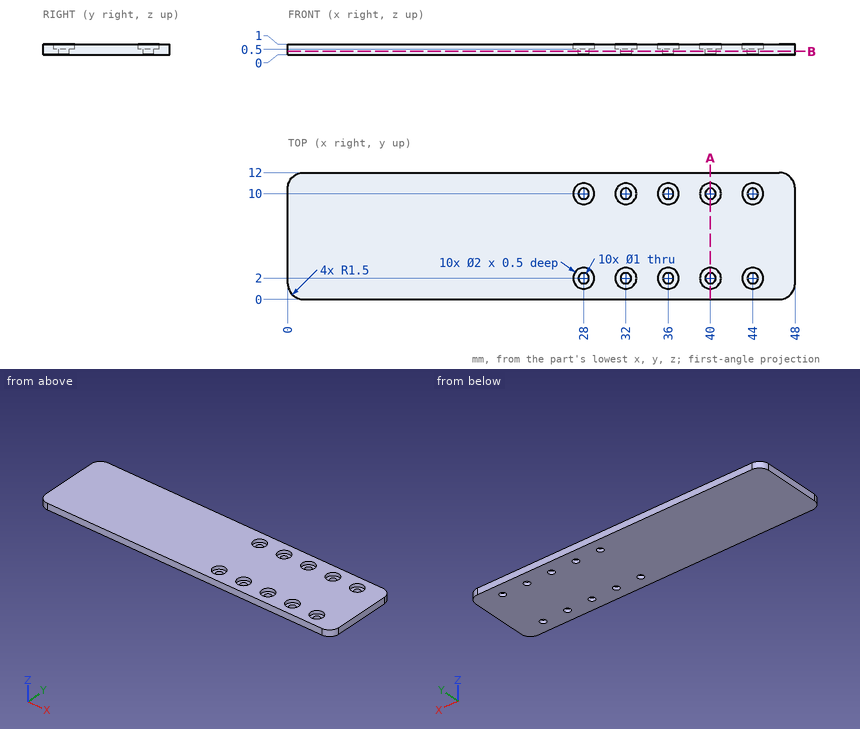
Study the drawing (mm; zero at the part's minimum x, y, z) and answer. Round coordinates to 2 decimals unless told otherwise and drop trailing zeros. Write each loop counter-clockwise with the first axis right and the second up, starting at its lowest first coordinate (ties: lowest second). Pieces come first, ordered by that corner, then holes. Notation, with made-up numbers: (78.5, 18.5) - (83.5, 18.5) arc R30 cw to (83.5, 55.5) - close; hole circle Ø4 at (-28.75, 11.5). An arc over 180 degrees is marked (long way). Return JSON: item names as keys, results as strings. Group by question number.
Q1. This flat-tipped pin is pushed along its axis until it touches: pin 1 Ø1.8 at (x, y) = (40, 10) entering from +Z. Where does it stop, or does it pass through?
Q2. The part is cut by section B-B on z = 0.3. Count the separate pieces of the cut face and the enclosed holes in it, then the cut area to 3 significant figures.
Q3. Find the intervals of material crossed by L1, parallel to Y at x = 40, z = 0.6; L2, parallel to Y at x = 44, z = 0.3; L3, parallel to X at y = 1.5, z = 0.9, in increasing order.
Q4. The part is cut by section A-A on x = 40. Write down the section's boundary in (y, z), then the cut area to 3 significant figures.
Solved:
{
 "1": {"pin 1": "z = 0.5"},
 "2": {"separate pieces": "1", "enclosed holes": "10", "area": "566 mm²"},
 "3": {"L1": "0 to 1, 3 to 9, 11 to 12", "L2": "0 to 1.5, 2.5 to 9.5, 10.5 to 12", "L3": "0 to 27.13, 28.87 to 31.13, 32.87 to 35.13, 36.87 to 39.13, 40.87 to 43.13, 44.87 to 48"},
 "4": {"outline": "(0, 0) - (1.5, 0) - (1.5, 0.5) - (1, 0.5) - (1, 1) - (0, 1) - close; (2.5, 0) - (9.5, 0) - (9.5, 0.5) - (9, 0.5) - (9, 1) - (3, 1) - (3, 0.5) - (2.5, 0.5) - close; (10.5, 0) - (12, 0) - (12, 1) - (11, 1) - (11, 0.5) - (10.5, 0.5) - close", "area": "9.00 mm²"}
}
